Autodesk Inventor part; units mm, degrees
ref_plane "YZ Plane" through (0, 0, 0) normal (1, 0, 0) x (0, 1, 0)
ref_plane "XZ Plane" through (0, 0, 0) normal (0, 1, 0) x (-1, 0, 0)
ref_plane "XY Plane" through (0, 0, 0) normal (0, 0, 1) x (1, 0, 0)
sketch "草圖1" plane through (0, 0, 0) normal (0, 0, 1) x (1, 0, 0)
  circle A0 centre (0, 0) radius 80
  circle A1 centre (0, 0) radius 70
  circle A2 centre (0, 0) radius 55
  dimension "d0" = 160
  dimension "d1" = 140
  dimension "d2" = 110
extrude "擠出1" add sketch "草圖1" against normal blind 30
sketch "草圖2" plane through (0, 0, -30) normal (0, 0, -1) x (-1, 0, 0)
  circle A0 centre (0, 0) radius 80
extrude "擠出2" add sketch "草圖2" along normal blind 10
sketch "草圖3" plane through (0, 0, -40) normal (0, 0, -1) x (-1, 0, 0)
  circle A0 centre (0, 0) radius 25
  dimension "d7" = 50
sketch "草圖4" plane through (0, 0, 0) normal (0, 0, 1) x (1, 0, 0)
  circle A0 centre (0, 0) radius 80
  circle A1 centre (0, 0) radius 70
  line L0 (0, 0) -> (-69.282, -40) construction
  line L1 (0, 0) -> (69.282, -40) construction
  line L2 (0, 0) -> (80, 0) construction
  line L3 (0, 0) -> (-80, 0) construction
  circle A2 centre (0, 0) radius 80
  line L4 (-69.282, -40) -> (-61.4878, -35.5)
  line L5 (69.282, -40) -> (61.4878, -35.5)
  circle A3 centre (0, 0) radius 70
  arc A4 (-61.4878, -35.5) -> (61.4878, -35.5) centre (0, 0) ccw
  dimension "d10" = 30
  dimension "d11" = 30
  dimension "d13" = 71
sketch "草圖5" plane through (0, 0, 0) normal (0, 1, 0) x (-1, 0, 0)
  line L0 (-59.2626, 395) -> (59.2626, 395) construction
  line L1 (0, 0) -> (0, 395) construction
  line L2 (66.7748, 395) -> (-66.7748, 395) construction
  line L3 (67.5187, 0) -> (67.5187, 395) construction
  line L4 (-67.5187, 0) -> (-67.5187, 395) construction
  arc A0 (67.5187, 375.1961) -> (-67.5187, 375.1961) centre (0, 270) ccw
  line L5 (67.5187, 375.1961) -> (67.5187, 415)
  line L6 (-67.5187, 375.1961) -> (-67.5187, 415)
  line L7 (-67.5187, 415) -> (67.5187, 415)
  dimension "d19" = 125
  dimension "d20" = 20
properties part number "螺旋鉤子底座"
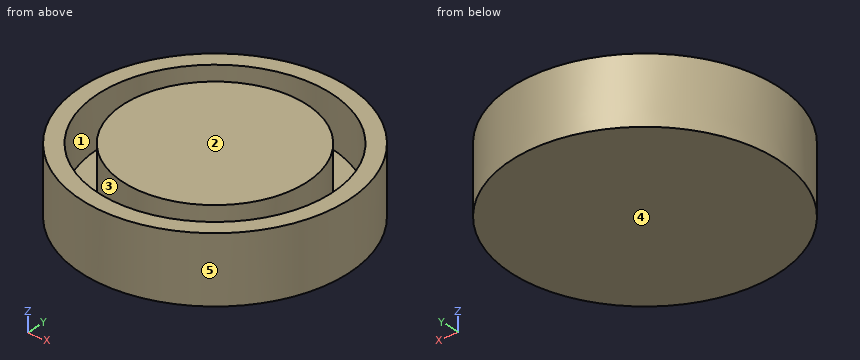
Here's how the part is built. I have some questions about the finished solid (model axes, mm). Face numbers are marked on the shaded views. A direction names the side the tool comes from. Coordinates: 2 decimals unless noted, no trailing zeros. Loops run counter-clockwise (first coordinate to the right, second up) from the corner with the lowest first, then second, coordinate; pieces in that order, holes last. Notation, with made-up numbers: (74, -21.5) - (126, -21.5) arc R12 cw to (126, -10.5) - close; hole circle Ø10 at (11, 1). An arc over 180 degrees is marked (long way). Return JSON: item names as keys, results as strings. Group by question number.
Item 1: If we section it at D-D on x = 68: Write out the boundary of the cut face in (y, z).
Item 2: If we section it at A-A on z = -17: Write out the boundary of the cut face in (x, y), and give its area (3 significant figures).
Item 3: If we section it at B-B on y = 0: Write out the boundary of the cut face in (x, z).
Item 4: Will these pins go through, and if not, where does the flat tip stop? P1, Ø3, axis at y = -14, z = -12.5, coming from the -X side; P2, Ø4, axis at y = -22, z = -8, coming from the +X side; P3, Ø8, axis at x = -44.5, z = -22, coming from the +Y side.
Item 5: On a 3-axis mill with a long thin cutter (end or side, diameter ignored), from which of +Z, -Z, +X, -X, +Y, -Y can I reach the whole of each face in a straight line? I mean the marked faces 1 and 2. Say none if no direction works.
Item 6: I need wall thicknesses on line 1 (Y direction, x = 0, z = -19); line 2 (Y direction, x = 43, z = -14); line 3 (X direction, y = -41.5, z = -24). Which ranges of each line are inside material? Lowest first, please. Write a range as from..to.
Item 7: We'd pull the mould along Y, two halves only. Please class the marked faces 3, 4 and 5: +Y half, -Y half, draft (parallel to the pull), parting line (faces both ways), or undercut.
Calculated:
{
 "1": {"outline": "(-42.14, -40) - (42.14, -40) - (42.14, 0) - (16.61, 0) - (16.61, -30) - (-16.61, -30) - (-16.61, 0) - (-42.14, 0) - close"},
 "2": {"outline": "circle Ø160 at (0, 0); circle Ø110 at (0, 0); hole circle Ø140 at (0, 0)", "area": "14,200 mm^2"},
 "3": {"outline": "(-80, -40) - (80, -40) - (80, 0) - (70, 0) - (70, -30) - (55, -30) - (55, 0) - (-55, 0) - (-55, -30) - (-70, -30) - (-70, 0) - (-80, 0) - close"},
 "4": {"P1": "stops at x = -79.02", "P2": "stops at x = 77.46", "P3": "stops at y = 68.99"},
 "5": {"face 1": "+Z", "face 2": "+Z, +X, -X, +Y, -Y"},
 "6": {"line 1": "y = -80..-70, -55..55, 70..80", "line 2": "y = -67.46..-55.24, -34.29..34.29, 55.24..67.46", "line 3": "x = -68.39..-56.37, -36.09..36.09, 56.37..68.39"},
 "7": {"face 3": "undercut", "face 4": "draft", "face 5": "parting line"}
}
